```python
from build123d import *

# Parameters (mm, degrees)
SKETCH1_R           = 63.5
BOSS_EXTRUDE1_DEPTH = 31.75
SKETCH2_R           = 57.15
SKETCH2_R_2         = 55.5625
CUT_EXTRUDE1_DEPTH  = 3.175


with BuildPart() as part:
    # Sketch1 → Boss-Extrude1 (new body)
    with BuildSketch(Plane.XY):
        Circle(SKETCH1_R)
    extrude(amount=BOSS_EXTRUDE1_DEPTH)

    # Sketch2 → Cut-Extrude1 (cut)
    with BuildSketch(Plane(origin=(0, 0, 0), x_dir=(-1, 0, 0), z_dir=(0, 0, -1))):
        Circle(SKETCH2_R)
        Circle(SKETCH2_R_2, mode=Mode.SUBTRACT)
    extrude(amount=-CUT_EXTRUDE1_DEPTH, mode=Mode.SUBTRACT)


solid = part.part
```
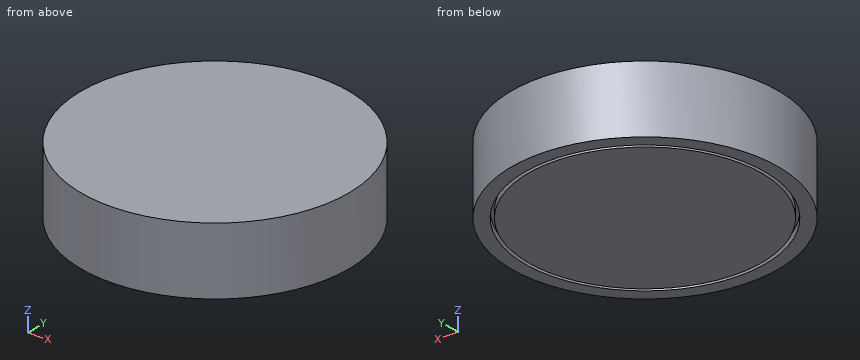
CAD build for the part. Positions are in the model's coordinates, mm. Coordinates: 2 decimals unless noted, no trailing zeros. Order: outer loops, then holes, each group sorted by start corner. A loop starts at its lowest first (then second) coordinate and runs counter-clockwise, first axis right, second up. Notation, with made-up numbers: (24, -14.5) - (81, -14.5) arc R33 cw to (81, 23.5) - close; hole circle Ø2 at (5, 49). An arc over 180 degrees is marked (long way). Use a Markdown table: item, result. Add a question column.
(1) Saw through at B-B (x = -22.5). Give the cut face in (y, z) (3 decimals).
(2) Flat gauge pins, fed straight in: pin 1 (4 mm diameter, centred on x = 9.5, z = 19, fed in from -Y); pin 2 (1 mm diameter, centred on x = 40.5, z = 19, fed in from -Y); pin 3 (10 mm diameter, centred on x = -34.5, z = 26.5, fed in from +Y). Where does each tip first touch, or does it go through?
(3) Drill centre lines: line 1 along Y through (x, z) = (0, 2.2); line 2 along X through (y, z) = (-34, 2.5); line 3 along X through (y, z) = (-39.5, 2). Where is each one in solid material? Low to high. Write a range as [from, to].
(4) Saw through at A-A (y = -11). Give the cut face in (x, z) (3 decimals).
Solved:
| question | item | result |
|---|---|---|
| 1 | outline | (-59.38, 0) - (-52.534, 0) - (-52.534, 3.175) - (-50.803, 3.175) - (-50.803, 0) - (50.803, 0) - (50.803, 3.175) - (52.534, 3.175) - (52.534, 0) - (59.38, 0) - (59.38, 31.75) - (-59.38, 31.75) - close |
| 2 | pin 1 | stops at y = -63.06 |
| 2 | pin 2 | stops at y = -49.32 |
| 2 | pin 3 | stops at y = 56.23 |
| 3 | line 1 | y = [-63.5, -57.15], [-55.56, 55.56], [57.15, 63.5] |
| 3 | line 2 | x = [-53.63, -45.94], [-43.95, 43.95], [45.94, 53.63] |
| 3 | line 3 | x = [-49.72, -41.3], [-39.08, 39.08], [41.3, 49.72] |
| 4 | outline | (-62.54, 0) - (-56.081, 0) - (-56.081, 3.175) - (-54.463, 3.175) - (-54.463, 0) - (54.463, 0) - (54.463, 3.175) - (56.081, 3.175) - (56.081, 0) - (62.54, 0) - (62.54, 31.75) - (-62.54, 31.75) - close |
